The listing builds one solid part. Answer for the finished solid, in the listing's coordinates (mm). Round coordinates to 2 decimals unless told otherwise and drop trailing zeros. One line per item, written item: value.
```python
from build123d import *

# Parameters (mm, degrees)
F2_T     = -1
F5_ANGLE = 30


with BuildPart() as f1:
    # F0 (on Front) → F1 (revolve)
    with BuildSketch(Plane.XZ):
        Polygon((10, 40), (0, 40), (0, 0), (25, 0), (12, 30), align=None)
    revolve(axis=Axis((0, 0, 20), (0, 0, 1)))

    # F2
    f2_openings = [f1.faces().sort_by_distance(p)[0] for p in [
        (0, 0, 0),
        (0, 0, 40),
    ]]
    offset(amount=F2_T, openings=f2_openings, kind=Kind.INTERSECTION)


with BuildPart() as f1_1:
    # F3: moved
    add(f1.part.moved(Location((30, 0, 50))))


with BuildPart() as f1_2:
    # F5: moved
    add(f1_1.part.rotate(Axis((30, 0, 90), (0, -1, 0)), F5_ANGLE))


solid = f1_2.part
```
1) Consider L1, parallel to X at y = 6, z = 71.5; L2, parallel to Y at x = 37.5, z = 50.5; L3, parallel to Y at x = 35.5, z = 69. Determine where each line is inside the solid, lowest interval first.
Final values:
L1: 26.32 to 27.42, 63.7 to 65.48
L2: -20.15 to -18.83, 18.83 to 20.15
L3: -15.73 to -14.56, 14.56 to 15.73
2) Each of these flat-tipped pins is pushed along its axis until it touches: pin 1 Ø5 at (y, z) = (-6.5, 78.5) entering from +X; pin 2 Ø1 at (y, z) = (-15, 66) entering from -X; pin 3 Ø2 at (y, z) = (5.5, 61) entering from -X. Where does it stop, or does it pass through?
Final values:
pin 1: x = 59.17
pin 2: x = 32.93
pin 3: x = 26.77
3) For a pull along Y with two mould halves and no side action, classify faces 1 (the conical face through (39.025, -3.653, 91.99)), 2 (the conical face through (29.19, -8.84, 68.35)), 3 (the conical face through (40.06, 3.17, 92.68)) as released by +Y, released by -Y, zero draft, split by the parting line, or undercut.
Final values:
face 1: undercut
face 2: undercut
face 3: split by the parting line
